```python
from build123d import *

# Parameters (mm, degrees)
BOSS_EXTRUDE1_DEPTH = 69.85
SKETCH2_R           = 2.0193
CUT_EXTRUDE1_DEPTH  = 5.064
SKETCH3_R           = 2.35585
SKETCH3_R_2         = 13.97
CUT_EXTRUDE2_DEPTH  = 5.064


with BuildPart() as part:
    # Sketch1 → Boss-Extrude1 (new body)
    with BuildSketch(Plane(origin=(0, 0, 0), x_dir=(1, 0, 0), z_dir=(0, 1, 0))):
        Polygon((0, 0), (50.8, 0), (50.8, 42.626261264), (46.736, 39.216160363), (46.736, 4.064), (4.8432866, 4.064), align=None)
    extrude(amount=BOSS_EXTRUDE1_DEPTH)

    # Sketch2 → Cut-Extrude1 (cut, through all)
    with BuildSketch(Plane.ZY.offset(-46.736)):
        with Locations((-34.340080181, 63.5)):
            Circle(SKETCH2_R)
        with Locations((-8.940080181, 63.5)):
            Circle(SKETCH2_R)
        with Locations((-8.940080181, 48.26)):
            Circle(SKETCH2_R)
        with Locations((-34.340080181, 48.26)):
            Circle(SKETCH2_R)
    extrude(amount=-CUT_EXTRUDE1_DEPTH, mode=Mode.SUBTRACT)

    # Sketch3 → Cut-Extrude2 (cut, through all)
    with BuildSketch(Plane(origin=(0, 0, -4.064), x_dir=(-1, 0, 0), z_dir=(0, 0, -1))):
        with Locations((-40.9956, 46.482)):
            Circle(SKETCH3_R)
        with Locations((-20.6756, 46.482)):
            Circle(SKETCH3_R)
        with Locations((-20.6756, 8.382)):
            Circle(SKETCH3_R)
        with Locations((-40.9956, 8.382)):
            Circle(SKETCH3_R)
        with Locations((-30.8356, 27.432)):
            Circle(SKETCH3_R_2)
    extrude(amount=-CUT_EXTRUDE2_DEPTH, mode=Mode.SUBTRACT)


solid = part.part
```
For this review, take the finished solid that the model builds, in its own axes (mm). A direction names the side the tool comes from. Round coordinates to 2 decimals unless told otherwise and drop trailing zeros. Order: outer loops, then holes, each group sorted by start corner. A loop starts at its lowest first (then second) coordinate and runs counter-clockwise, first axis right, second up.
Q1. We need section C-C, the plane x = 10. Give the boundary of the cut face in (y, z), plus the area to 3 significant figures.
Findings below:
outline: (0, -4.06) - (69.85, -4.06) - (69.85, 0) - (0, 0) - close
area: 284 mm2
Q2. Mouldability with a two-part tool opening along X and no side actions: class faces 3 (the cylindrical face through (48.74, 65.502, -34.603)), 4 (the cylindrical face through (43.35, 8.49, -2.06)), 5 (the flat face through (48.8, 34.44, -40.95)) as pulls with the +X half, pulls with the -X half, needs draft (parallel to the pull), parting line crosses it, or undercut.
Findings below:
face 3: needs draft
face 4: undercut
face 5: pulls with the -X half
Q3. We need section B-B, the plane y = 18.5. Give the boundary of the cut face in (x, z), plus the area to 3 significant figures.
Findings below:
outline: (0, 0) - (4.84, -4.06) - (20.09, -4.06) - (20.09, 0) - close; (41.58, -4.06) - (46.74, -4.06) - (46.74, -39.22) - (50.8, -42.63) - (50.8, 0) - (41.58, 0) - close
area: 259 mm2
Q4. Insertion check: P1, Ø8, axis at x = 17, z = -8, coming from the -Y side; P2, Ø5.5, axis at y = 63.5, z = -8.94, coming from the -X side; P3, Ø12, axis at x = 39, y = 48.5, coming from the -Z side; P4, Ø8, axis at x = 43.5, y = 8, coming from the -Z side. Each pin has a flat end and moves straight along its axis. Give the tip position at first contact, or say it passes through.
Findings below:
P1: stops at y = 0
P2: stops at x = 46.74
P3: stops at z = -4.06
P4: stops at z = -39.86
Q5. Machinability: for faces 1 (the cylindrical face through (19.41, 48.47, -2.06)), 2 (the flat face through (46.736, 34, -22)), which of the approach directions +Z, -Z, +X, -X, +Y, -Y give a long, thin tool a straight path to every point of the face, cutting with its end or side? Answer none if there is none.
Findings below:
face 1: +Z, -Z
face 2: -Z, -X, +Y, -Y
Q6. Wall thickness on line 1 (Y direction, x = 20, z = -3); line 2 (X direction, y = 24, z = -33.5); line 3 (Z direction, x = 12.5, y = 7): over which ranges is each line inside the solid? List them lowest first.
Findings below:
line 1: y = 0 to 6.13, 10.64 to 18.61, 36.25 to 44.23, 48.74 to 69.85
line 2: x = 46.74 to 50.8
line 3: z = -4.06 to 0
Q7. We need section A-A, the plane y = 63.5. Give the boundary of the cut face in (x, z).
Findings below:
outline: (0, 0) - (4.84, -4.06) - (46.74, -4.06) - (46.74, -6.92) - (50.8, -6.92) - (50.8, 0) - close; (46.74, -39.22) - (50.8, -42.63) - (50.8, -36.36) - (46.74, -36.36) - close; (46.74, -32.32) - (50.8, -32.32) - (50.8, -10.96) - (46.74, -10.96) - close
Q8. We need section D-D, the plane z = -20. Give the boundary of the cut face in (x, y), plus the area to 3 significant figures.
Findings below:
outline: (46.74, 0) - (50.8, 0) - (50.8, 69.85) - (46.74, 69.85) - close
area: 284 mm2
